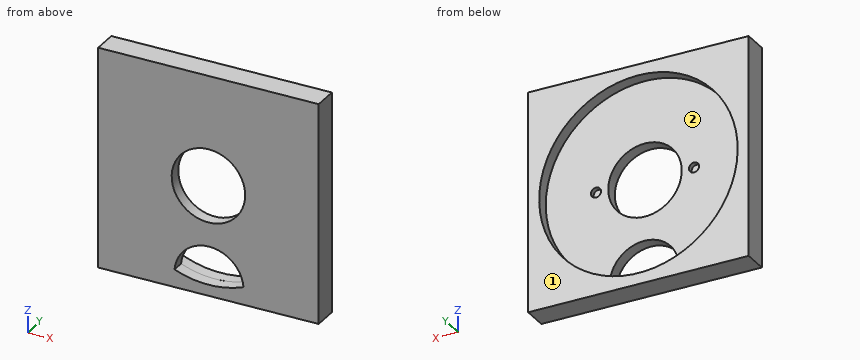
```python
from build123d import *

# Parameters (mm, degrees)
BOSS_EXTRUDE1_DEPTH = 10
SKETCH2_R           = 40.5
CUT_EXTRUDE1_DEPTH  = 5
SKETCH4_R           = 2.05
CUT_EXTRUDE2_DEPTH  = 2
SKETCH5_R           = 15
CUT_EXTRUDE3_DEPTH  = 64.835726674
CUT_EXTRUDE4_DEPTH  = 36


with BuildPart() as part:
    # Sketch1 → Boss-Extrude1 (new body)
    with BuildSketch(Plane(origin=(0, 0, 0), x_dir=(1, 0, 0), z_dir=(0, 1, 0))):
        Polygon((0, -45), (-45, -45), (-45, 45), (0, 45), (45, 45), (45, -45), align=None)
    extrude(amount=BOSS_EXTRUDE1_DEPTH)

    # Sketch2 → Cut-Extrude1 (cut)
    with BuildSketch(Plane(origin=(0, 10, 0), x_dir=(1, 0, 0), z_dir=(0, 1, 0))):
        with Locations(Location((0, 0, 0), (0, 0, 270))):
            Circle(SKETCH2_R)
    extrude(amount=-CUT_EXTRUDE1_DEPTH, mode=Mode.SUBTRACT)

    # Sketch4 → Cut-Extrude2 (cut)
    with BuildSketch(Plane(origin=(0, 5, 0), x_dir=(1, 0, 0), z_dir=(0, 1, 0))):
        with Locations(Location((-20, 0, 0), (0, 0, 270))):
            Circle(SKETCH4_R)
        with Locations(Location((20, 0, 0), (0, 0, 270))):
            Circle(SKETCH4_R)
    extrude(amount=-CUT_EXTRUDE2_DEPTH, mode=Mode.SUBTRACT)

    # Sketch5 → Cut-Extrude3 (cut, through all)
    with BuildSketch(Plane(origin=(0, 5, 0), x_dir=(1, 0, 0), z_dir=(0, 1, 0))):
        with Locations(Location((0, 0, 0), (0, 0, 270))):
            Circle(SKETCH5_R)
    extrude(amount=-CUT_EXTRUDE3_DEPTH, mode=Mode.SUBTRACT)

    # Sketch7 → Cut-Extrude4 (cut)
    with BuildSketch(Plane(origin=(0, 5, 0), x_dir=(1, 0, 0), z_dir=(0, 1, 0))):
        with BuildLine():
            ThreePointArc((-13.841521615, 37.800491998), (0.234545088, 24.817118498), (14.31061179, 37.800491998))
            ThreePointArc((14.31061179, 37.800491998), (0.234545088, 40.503688372), (-13.841521615, 37.800491998))
        make_face()
    extrude(amount=-CUT_EXTRUDE4_DEPTH, mode=Mode.SUBTRACT)


solid = part.part
```
Model file for the job. Use its own axes, mm. Face numbers are marked on the shaded views. A direction names the side the tool comes from. Round coordinates to 2 decimals unless told otherwise and drop trailing zeros. Write each loop counter-clockwise with the first axis right and the second up, starting at its lowest first coordinate (ties: lowest second). Pieces come first, ordered by that corner, then holes. Notation, with made-up numbers: M 41,10.5 L 86,10.5 A18 cw 86,31.5 Z; hole C 57.5,-38 d9. An arc over 180 degrees is marked long. Put each result on its own line as item: value.
Item 1: Cut at A-A (z = 0). List the corners of the cut face in (x, y).
Responses:
outline: M -45,0 L -15,0 L -15,5 L -17.95,5 L -17.95,3 L -22.05,3 L -22.05,5 L -40.5,5 L -40.5,10 L -45,10 Z; M 15,0 L 45,0 L 45,10 L 40.5,10 L 40.5,5 L 22.05,5 L 22.05,3 L 17.95,3 L 17.95,5 L 15,5 Z
Item 2: Probe L1, parallel to X at y = 6.25, z = 0.5; L2, parallel to Z at x = 3.5, y = 3.5; L3, parallel to X at y = 8.25, z = 15.5. List the from-to ranges inside material, lowest first. Write a range as from..to.
Responses:
L1: -45..-40.5, 40.5..45
L2: -45..-40.36, -25.2..-14.59, 14.59..45
L3: -45..-37.42, 37.42..45
Item 3: Tool access for the marked faces 1 and 2: list every direction of +Z, -Z, +X, -X, +Y, -Y with a clear straight run to the whole face (end or side of a thin tool).
Responses:
face 1: +Z, -Z, +X, -X, +Y
face 2: +Y
Item 4: Cut at B-B (y = 8.75). List the corners of the cut face in (x, z).
Responses:
outline: M -45,-45 L 45,-45 L 45,45 L -45,45 Z; hole C 0,0 d81
Item 5: Cut at C-C (x = 20). List the corners of the cut face in (y, z), and give its area (3 significant figures).
Responses:
outline: M 0,-45 L 10,-45 L 10,-35.22 L 5,-35.22 L 5,-2.05 L 3,-2.05 L 3,2.05 L 5,2.05 L 5,35.22 L 10,35.22 L 10,45 L 0,45 Z
area: 540 mm²
Item 6: Cut at D-D (z = 32). List the corners of the cut face in (x, y).
Responses:
outline: M -45,0 L 45,0 L 45,10 L 24.82,10 L 24.82,5 L -24.82,5 L -24.82,10 L -45,10 Z
Item 7: Flat gauge pins, fed straight in: P1, Ø3.5, axis at x = 20, z = 0, coming from the +Y side; P2, Ø3.5, axis at x = 19.5, z = -0.5, coming from the +Y side. Where does each tip first touch, or does it go through?
Responses:
P1: y = 3
P2: y = 5
